Autodesk Inventor part; units mm, degrees
ref_plane "YZ Plane" through (0, 0, 0) normal (1, 0, 0) x (0, 1, 0)
ref_plane "XZ Plane" through (0, 0, 0) normal (0, 1, 0) x (-1, 0, 0)
ref_plane "XY Plane" through (0, 0, 0) normal (0, 0, 1) x (1, 0, 0)
sketch "Sketch1" plane through (0, 0, 0) normal (0, 0, 1) x (1, 0, 0)
  line L0 (13.5, -39.75) -> (11.5, -39.75)
  arc A0 (11.5, -39.75) -> (9.25, -42) centre (11.5, -42) ccw
  line L1 (9.25, -42) -> (9.25, -44)
  arc A1 (8.25, -45) -> (9.25, -44) centre (8.25, -44) ccw
  line L2 (8.25, -45) -> (-8.25, -45)
  arc A2 (-9.25, -44) -> (-8.25, -45) centre (-8.25, -44) ccw
  line L3 (-9.25, -44) -> (-9.25, -42)
  arc A3 (-9.25, -42) -> (-11.5, -39.75) centre (-11.5, -42) ccw
  line L4 (-11.5, -39.75) -> (-13.5, -39.75)
  arc A4 (-14.5, -38.75) -> (-13.5, -39.75) centre (-13.5, -38.75) ccw
  line L5 (-14.5, -38.75) -> (-14.5, 8.25)
  arc A5 (-13.5, 9.25) -> (-14.5, 8.25) centre (-13.5, 8.25) ccw
  line L6 (-13.5, 9.25) -> (-11.5, 9.25)
  arc A6 (-11.5, 9.25) -> (-9.25, 11.5) centre (-11.5, 11.5) ccw
  line L7 (-9.25, 11.5) -> (-9.25, 14.5)
  line L8 (-15, 14.5) -> (-9.25, 14.5)
  line L9 (-20.1, 8.5) -> (-15, 14.5)
  line L10 (-20.1, -44.6) -> (-20.1, 8.5)
  line L11 (-15, -50.6) -> (-20.1, -44.6)
  line L12 (15, -50.6) -> (-15, -50.6)
  line L13 (20.1, -44.6) -> (15, -50.6)
  line L14 (20.1, 8.5) -> (20.1, -44.6)
  line L15 (15, 14.5) -> (20.1, 8.5)
  line L16 (9.25, 14.5) -> (15, 14.5)
  line L17 (9.25, 14.5) -> (9.25, 11.5)
  arc A7 (9.25, 11.5) -> (11.5, 9.25) centre (11.5, 11.5) ccw
  line L18 (11.5, 9.25) -> (13.5, 9.25)
  arc A8 (14.5, 8.25) -> (13.5, 9.25) centre (13.5, 8.25) ccw
  line L19 (14.5, 8.25) -> (14.5, -38.75)
  arc A9 (13.5, -39.75) -> (14.5, -38.75) centre (13.5, -38.75) ccw
  circle A10 centre (17.3, 4) radius 1.35
  circle A11 centre (17.3, -18) radius 1.35
  circle A12 centre (11, -47.8) radius 1.35
  circle A13 centre (-17.3, 4) radius 1.35
  circle A14 centre (-17.3, -18) radius 1.35
  circle A15 centre (-11, -47.8) radius 1.35
  circle A16 centre (17.3, -40) radius 1.35
  circle A17 centre (-17.3, -40) radius 1.35
  point P0 (0, 0)
extrude "Extrusion1" add sketch "Sketch1" along normal blind 10
sketch "Sketch2" plane through (-15, -50.6, 0) normal (0, -1, 0) x (1, 0, 0)
  line L0 (0, 0) -> (30, 0)
  line L1 (30, 0) -> (30, 10)
  line L2 (0, 10) -> (30, 10)
  line L3 (0, 0) -> (0, 10)
  line L4 (15, 0) -> (70, 0)
  line L5 (70, 0) -> (70, 10)
  line L6 (70, 10) -> (15, 10)
  line L7 (15, 10) -> (15, 0)
  line L8 (15, 0) -> (-40, 0)
  line L9 (-40, 0) -> (-40, 10)
  line L10 (-40, 10) -> (15, 10)
  line L11 (15, 10) -> (15, 0)
  dimension "d2" = 55
  dimension "d3" = 10
  dimension "d4" = 55
  dimension "d5" = 10
extrude "Extrusion2" add sketch "Sketch2" along normal blind 10
sketch "Sketch3" plane through (0, 0, 10) normal (0, 0, 1) x (1, 0, 0)
  circle A0 centre (-17.3, -40) radius 1.35
  circle A1 centre (17.3, -40) radius 1.35
  circle A2 centre (-11, -47.8) radius 1.35
  circle A3 centre (-17.3, -18) radius 1.35
  circle A4 centre (-17.3, 4) radius 1.35
  circle A5 centre (11, -47.8) radius 1.35
  circle A6 centre (17.3, -18) radius 1.35
  circle A7 centre (17.3, 4) radius 1.35
  line L0 (13.5, -39.75) -> (11.5, -39.75)
  arc A8 (11.5, -39.75) -> (9.25, -42) centre (11.5, -42) ccw
  line L1 (9.25, -42) -> (9.25, -44)
  arc A9 (8.25, -45) -> (9.25, -44) centre (8.25, -44) ccw
  line L2 (8.25, -45) -> (-8.25, -45)
  arc A10 (-9.25, -44) -> (-8.25, -45) centre (-8.25, -44) ccw
  line L3 (-9.25, -44) -> (-9.25, -42)
  arc A11 (-9.25, -42) -> (-11.5, -39.75) centre (-11.5, -42) ccw
  line L4 (-11.5, -39.75) -> (-13.5, -39.75)
  arc A12 (-14.5, -38.75) -> (-13.5, -39.75) centre (-13.5, -38.75) ccw
  line L5 (-14.5, -38.75) -> (-14.5, 8.25)
  arc A13 (-13.5, 9.25) -> (-14.5, 8.25) centre (-13.5, 8.25) ccw
  line L6 (-13.5, 9.25) -> (-11.5, 9.25)
  arc A14 (-11.5, 9.25) -> (-9.25, 11.5) centre (-11.5, 11.5) ccw
  line L7 (-9.25, 11.5) -> (-9.25, 14.5)
  line L8 (-9.25, 14.5) -> (-15, 14.5)
  line L9 (-15, 14.5) -> (-20.1, 8.5)
  line L10 (-20.1, 8.5) -> (-20.1, -44.6)
  line L11 (-20.1, -44.6) -> (-15, -50.6)
  line L12 (-15, -50.6) -> (-55, -50.6)
  line L13 (-55, -50.6) -> (-55, -60.6)
  line L14 (55, -60.6) -> (-55, -60.6)
  line L15 (55, -50.6) -> (55, -60.6)
  line L16 (55, -50.6) -> (15, -50.6)
  line L17 (15, -50.6) -> (20.1, -44.6)
  line L18 (20.1, -44.6) -> (20.1, 8.5)
  line L19 (20.1, 8.5) -> (15, 14.5)
  line L20 (15, 14.5) -> (9.25, 14.5)
  line L21 (9.25, 14.5) -> (9.25, 11.5)
  arc A15 (9.25, 11.5) -> (11.5, 9.25) centre (11.5, 11.5) ccw
  line L22 (11.5, 9.25) -> (13.5, 9.25)
  arc A16 (14.5, 8.25) -> (13.5, 9.25) centre (13.5, 8.25) ccw
  line L23 (14.5, 8.25) -> (14.5, -38.75)
  arc A17 (13.5, -39.75) -> (14.5, -38.75) centre (13.5, -38.75) ccw
  line L24 (-20.1, 8.5) -> (-55, -50.6)
  line L25 (20.1, -44.6) -> (20.1, 8.5)
  line L26 (15, -50.6) -> (55, -50.6)
  line L27 (20.1, 8.5) -> (55, -50.6)
  point P0 (0, 0)
extrude "Extrusion3" add sketch "Sketch3" against normal blind 10 contours L27 L16 L17 L18 | L24 L10 L11 L12
sketch "Sketch4" plane through (-15, -60.6, 0) normal (0, -1, 0) x (1, 0, 0)
  line L0 (15, 0) -> (15, 5)
  line L1 (15, 0) -> (20, 0) construction
  line L2 (15, 5) -> (-35, 5)
  line L3 (15, 5) -> (65, 5)
  line L4 (15, 5) -> (65, 5) construction
  circle A0 centre (-35, 5) radius 2.1
  circle A1 centre (65, 5) radius 2.1
  dimension "d10" = 5
  dimension "d11" = 90
  dimension "d12" = 50
  dimension "d13" = 90
  dimension "d14" = 50
  dimension "d15" = 0
  dimension "d16" = 4.2
  dimension "d17" = 4.2
extrude "Extrusion4" cut sketch "Sketch4" against normal blind 10
ref_plane "Work Plane1" through (-15, -55.6, 0) normal (0, -1, 0) x (1, 0, 0)
sketch "Sketch5" plane through (-15, -55.6, 0) normal (0, -1, 0) x (1, 0, 0)
  circle A0 centre (-35, 5) radius 2.1
  circle A1 centre (65, 5) radius 2.1
  line L0 (-38.6, 8.6) -> (-31.4, 8.6)
  line L1 (-31.4, 8.6) -> (-31.4, 1.4)
  line L2 (-31.4, 1.4) -> (-38.6, 1.4)
  line L3 (-38.6, 1.4) -> (-38.6, 8.6)
  line L4 (-38.6, 8.6) -> (-31.4, 1.4)
  line L5 (-31.4, 8.6) -> (-38.6, 1.4)
  line L6 (61.4, 8.6) -> (68.6, 8.6)
  line L7 (68.6, 8.6) -> (68.6, 1.4)
  line L8 (68.6, 1.4) -> (61.4, 1.4)
  line L9 (61.4, 1.4) -> (61.4, 8.6)
  line L10 (61.4, 8.6) -> (68.6, 1.4)
  line L11 (68.6, 8.6) -> (61.4, 1.4)
  line L12 (70, 0) -> (70, 10)
  line L13 (68.6, 1.4) -> (70, 1.4)
  line L14 (70, 1.4) -> (70, 8.6)
  line L15 (70, 8.6) -> (68.6, 8.6)
  line L16 (68.6, 8.6) -> (68.6, 1.4)
  line L17 (-40, 10) -> (-40, 0) construction
  line L18 (-38.6, 8.6) -> (-40, 8.6)
  line L19 (-40, 8.6) -> (-40, 1.4)
  line L20 (-40, 1.4) -> (-38.6, 1.4)
  line L21 (-38.6, 1.4) -> (-38.6, 8.6)
  point P0 (15, 0)
  dimension "d21" = 7.2
  dimension "d22" = 7.2
  dimension "d23" = 7.2
  dimension "d24" = 7.2
extrude "Extrusion5" cut sketch "Sketch5" against normal blind 2.5
properties part number "motor_mount"
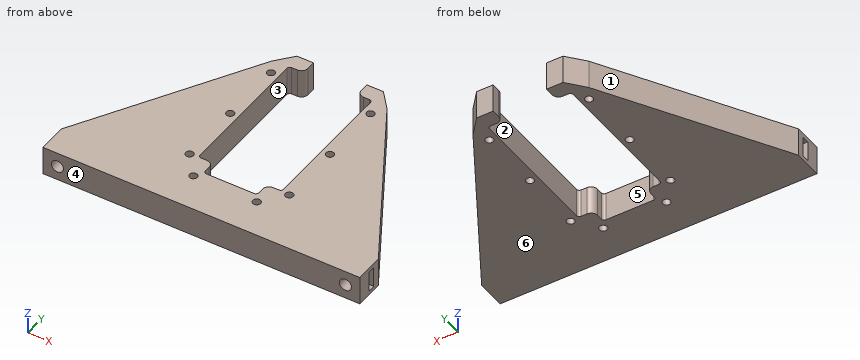
CAD build for the part. Positions are in the model's coordinates, mm. Face numbers are marked on the shaded views. A direction names the side the tool comes from. Coordinates: 2 decimals unless noted, no trailing zeros. Order: outer loops, then holes, each group sorted by start corner. A loop starts at its lowest first (then second) coordinate and runs counter-clockwise, first axis right, second up. Notation, with made-up numbers: (-40, -30.75) - (-22, -30.75) arc R8 cw to (-22, -22.75) - close; hole circle Ø6 at (-31.5, -29.5). An arc over 180 degrees is marked (long way). Use a Markdown table: item, result. Add a question column.
(1) Drill centre lines: line 1 along Z through (x, y) = (-50, -51.4); line 2 along X through (y, z) = (-39.5, 9.25); line 3 along X through (y, z) = (-57, 3.25). Where is each one in solid material? Low to high. Write a range as [from, to].
(2) Which spindle directions (+Z, -Z, +X, -X, +Y, -Y) get a long thin tool onto all of the face, cutting with end or side? Do the marked faces 5 and 6. Say none if no direction does.
(3) Flat gauge pins, fed straight in: pin 1 (2 mm diameter, centred on x = 11, y = -47.8, fed in from -Z); pin 2 (2 mm diameter, centred on x = 24, z = 8, fed in from +Y); pin 3 (2.5 mm diameter, centred on x = -50, z = 5, fed in from +Y); pin 4 (3 mm diameter, centred on y = -41.5, z = 8.5, fed in from +X). Where does each tip first touch, or does it go through?
(4) Pull direction Y, two halves, no side cores. Call the marked faces 1, 2, 3 and 4: +Y half, -Y half, draft (parallel to the pull), parting line (faces both ways), or undercut.
(5) Saw through at B-B (x = 17.3). Give the cut face in (y, z).
(6) Saw through at C-C (z = 5). Count the separate pieces of the cut face and the enclosed holes in it, then the cut area to 3 significant figures.
(7) Saw through at D-D (y = -18). Give the cut face in (x, z).
(8) Saw through at A-A (y = -28). Give the cut face in (x, z).
Solved:
| question | item | result |
|---|---|---|
| 1 | line 1 | z = [0, 2.9], [7.1, 10] |
| 1 | line 2 | x = [-48.45, -18.55], [-16.05, -14.16], [14.16, 16.05], [18.55, 48.45] |
| 1 | line 3 | x = [-55, -51.16], [-48.84, 48.84], [51.16, 55] |
| 2 | face 5 | +Z, -Z, +Y |
| 2 | face 6 | -Z, +X, -X, +Y, -Y |
| 3 | pin 1 | passes through |
| 3 | pin 2 | stops at y = 3.59 |
| 3 | pin 3 | stops at y = -40.02 |
| 3 | pin 4 | stops at x = 50.51 |
| 4 | face 1 | +Y half |
| 4 | face 2 | undercut |
| 4 | face 3 | undercut |
| 4 | face 4 | -Y half |
| 5 | outline | (-60.6, 0) - (-41.35, 0) - (-41.35, 10) - (-60.6, 10) - close; (-38.65, 0) - (-19.35, 0) - (-19.35, 10) - (-38.65, 10) - close; (-16.65, 0) - (2.65, 0) - (2.65, 10) - (-16.65, 10) - close; (5.35, 0) - (11.79, 0) - (11.79, 10) - (5.35, 10) - close |
| 6 | separate pieces | 3 |
| 6 | enclosed holes | 8 |
| 6 | area | 3,980 mm² |
| 7 | outline | (-35.75, 0) - (-18.65, 0) - (-18.65, 10) - (-35.75, 10) - close; (-15.95, 0) - (-14.5, 0) - (-14.5, 10) - (-15.95, 10) - close; (14.5, 0) - (15.95, 0) - (15.95, 10) - (14.5, 10) - close; (18.65, 0) - (35.75, 0) - (35.75, 10) - (18.65, 10) - close |
| 8 | outline | (-41.65, 0) - (-14.5, 0) - (-14.5, 10) - (-41.65, 10) - close; (14.5, 0) - (41.65, 0) - (41.65, 10) - (14.5, 10) - close |
